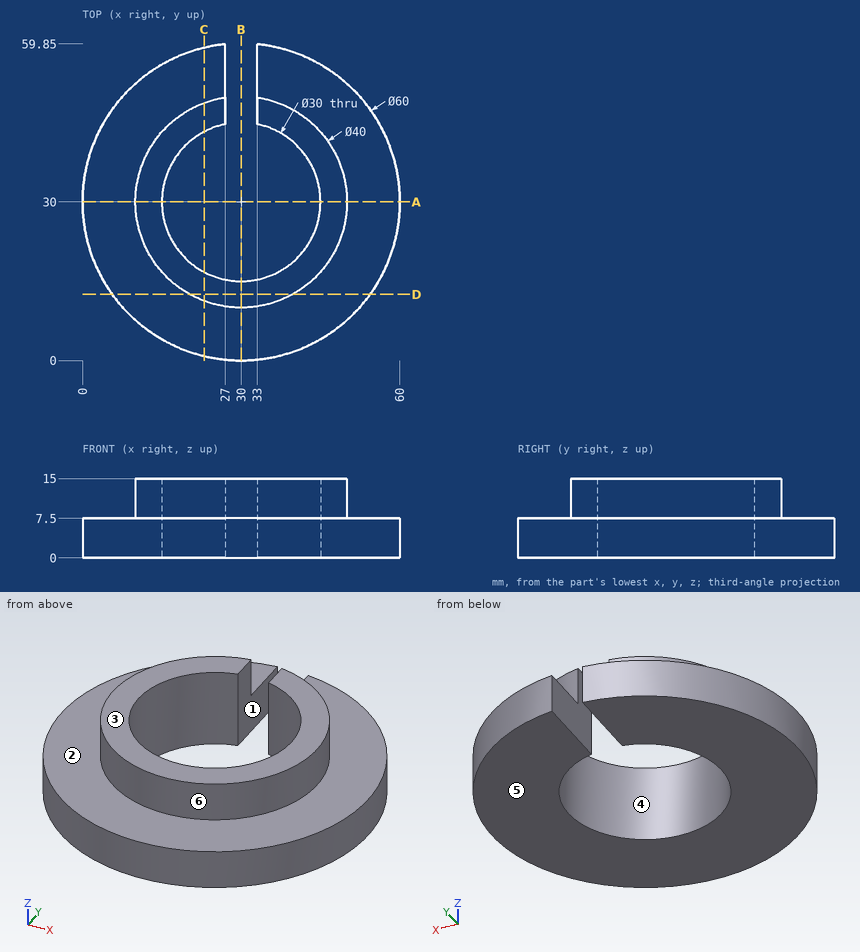
Input: dimensioned drawing with shaded views. Units: mm. Origin: part minimum x, y, z. A direction names the side the tool comes from. Coordinates: 2 decimals unless noted, no trailing zeros. Order: outer loops, then holes, each group sorted by start corner. A loop starts at its lowest first (then second) coordinate and runs counter-clockwise, first axis right, second up.
(1) Draft query along X for the marked faces 4, 5 and 6. Return one class per face: pulls with the +X half, pulls with the -X half, needs draft (parallel to the pull), parting line crosses it, or undercut.
(2) Section query A-A (y = 30). Return the cut outline in (x, z), plus the area to 3 significant figures.
(3) Section query B-B (x = 30). Return the cut outline in (y, z).
(4) Section query C-C (x = 23). Return the cut outline in (y, z) (1 decimal).
(5) Access query for the marked faces 1, 2 and 3. Directions: +Z, -Z, +X, -X, +Y, -Y. A direction counts if a zero-diameter tool reaches every point of the face in a straight line with its end or side. Return the directions, or none.
(6) First-contact query: pin 1 (8 mm diameter, centred on y = 20.5, z = 6.5, fed in from -X); pin 2 (7.5 mm diameter, centred on y = 50.5, z = 8, fed in from +X) (1 decimal); pin 3 (2 mm diameter, centred on y = 23, z = 2, fed in from -X); pin 4 (2 mm diameter, centred on x = 28.5, y = 15.5, fed in from -Z). Flat tips, straight axial feed; report the tip coordinate or a pass-through.
(7) Section query D-D (y = 12.5). Return the cut outline in (x, z), plus the area to 3 significant figures.
(8) Material intervals for probe 1 along X at (y, z) = (30, 5); probe 2 along X at (y, z) = (30, 10.75); probe 3 along Y at (x, z) = (30, 12.25), sorted ascending.
Solution:
1. face 4: undercut
1. face 5: needs draft
1. face 6: parting line crosses it
2. outline: (0, 0) - (15, 0) - (15, 15) - (10, 15) - (10, 7.5) - (0, 7.5) - close; (45, 0) - (60, 0) - (60, 7.5) - (50, 7.5) - (50, 15) - (45, 15) - close
2. area: 300 mm2
3. outline: (0, 0) - (15, 0) - (15, 15) - (10, 15) - (10, 7.5) - (0, 7.5) - close
4. outline: (0.8, 0) - (16.7, 0) - (16.7, 15) - (11.3, 15) - (11.3, 7.5) - (0.8, 7.5) - close; (43.3, 0) - (59.2, 0) - (59.2, 7.5) - (48.7, 7.5) - (48.7, 15) - (43.3, 15) - close
5. face 1: +Z, -Z, +Y
5. face 2: +Z
5. face 3: +Z, +X, -X, +Y, -Y
6. pin 1: stops at x = 0.51
6. pin 2: stops at x = 54.9
6. pin 3: stops at x = 0.61
6. pin 4: stops at z = 0
7. outline: (5.63, 0) - (54.37, 0) - (54.37, 7.5) - (39.68, 7.5) - (39.68, 15) - (20.32, 15) - (20.32, 7.5) - (5.63, 7.5) - close
7. area: 511 mm2
8. probe 1: x = 0 to 15, 45 to 60
8. probe 2: x = 10 to 15, 45 to 50
8. probe 3: y = 10 to 15
